Verification items for the finished model (mm, model axes). A direction names the side the tool comes from. Coordinates: 2 decimals unless noted, no trailing zeros. Write each loop counter-clockwise with the first axis right and the second up, starting at its lowest first coordinate (ties: lowest second). Pieces come first, ordered by that corner, then holes.
```python
from build123d import *

# Parameters (mm, degrees)
F0_W     = 120
F0_H     = 37.7
F1_DEPTH = 2
F2_W     = 25
F2_H     = 8
F3_DEPTH = 25
F4_R     = 7.5
F5_R     = 2


with BuildPart() as f1:
    # F0 (on Top) → F1 (new body)
    with BuildSketch(Plane.XY):
        Rectangle(F0_W, F0_H)
    extrude(amount=F1_DEPTH)

    # F2 (on face) → F3 (cut)
    with BuildSketch(Plane.XY.offset(2)):
        with Locations((0, 18.85)):
            Rectangle(F2_W, F2_H)
        with Locations((0, -18.85)):
            Rectangle(F2_W, F2_H)
    extrude(amount=-F3_DEPTH, mode=Mode.SUBTRACT)

    # F4
    f4_edges = [f1.edges().sort_by_distance(p)[0] for p in [
        (-60, -18.85, 1),
        (60, -18.85, 1),
        (60, 18.85, 1),
        (-60, 18.85, 1),
    ]]
    fillet(f4_edges, radius=F4_R)

    # F5
    f5_edges = [f1.edges().sort_by_distance(p)[0] for p in [
        (-12.5, 14.85, 1),
        (12.5, 14.85, 1),
        (-12.5, -14.85, 1),
        (12.5, -14.85, 1),
    ]]
    fillet(f5_edges, radius=F5_R)


solid = f1.part
```
1. Gauge pin test, flat ends, axial feed: P1, Ø1, axis at y = 18.5, z = 0.5, coming from the -X side; P2, Ø1, axis at y = -18, z = 0.5, coming from the -X side; P3, Ø1, axis at x = 4.5, z = 1, coming from the +Y side. Record the tip position at first contact, or that the pin passes through.
2. Sectioned sample at A-A, the plane z = 1.55. Record the boundary of the cut face in (x, y).
3. Draft check along X on faces 4 (the flat face through (-1, 0, 2)), 5 (the flat face through (60, 0, 1)), 6 (the flat face through (-12.5, 18, 1)). Enter one of: pulls with the +X half, pulls with the -X half, needs draft (parallel to the pull), parting line crosses it, or undercut.
4. Material ranges on L1, parallel to Y at x = -2.5, z = 0.55; L2, parallel to X at y = -15.5, z = 1.35; L3, parallel to Y at x = 53, z = 0.3, recorded low to high.
5. Tool access check on faces 1 (the flat face through (12.5, -18, 1)), 2 (the cylindrical face through (-57.861, 16.595, 1.014)), 3 (the flat face through (0, 14.85, 1)). Record the directions out of +Z, -Z, +X, -X, +Y, -Y that give a thin tool (end or side, any length) a straight path to the whole face; none if there is none.
6. Sectioned sample at B-B, the plane x = -6. Record the boundary of the cut face in (y, z).
Outcome:
1. P1: stops at x = -55.97
1. P2: stops at x = -56.79
1. P3: stops at y = 14.85
2. outline: (-60, -11.35) arc R7.5 ccw to (-52.5, -18.85) - (-12.5, -18.85) - (-12.5, -16.85) arc R2 cw to (-10.5, -14.85) - (10.5, -14.85) arc R2 cw to (12.5, -16.85) - (12.5, -18.85) - (52.5, -18.85) arc R7.5 ccw to (60, -11.35) - (60, 11.35) arc R7.5 ccw to (52.5, 18.85) - (12.5, 18.85) - (12.5, 16.85) arc R2 cw to (10.5, 14.85) - (-10.5, 14.85) arc R2 cw to (-12.5, 16.85) - (-12.5, 18.85) - (-52.5, 18.85) arc R7.5 ccw to (-60, 11.35) - close
3. face 4: needs draft
3. face 5: pulls with the +X half
3. face 6: undercut
4. L1: y = -14.85 to 14.85
4. L2: x = -58.75 to -11.98, 11.98 to 58.75
4. L3: y = -18.83 to 18.83
5. face 1: +Z, -Z, -Y
5. face 2: +Z, -Z, -X, +Y
5. face 3: +Z, -Z, +Y
6. outline: (-14.85, 0) - (14.85, 0) - (14.85, 2) - (-14.85, 2) - close
